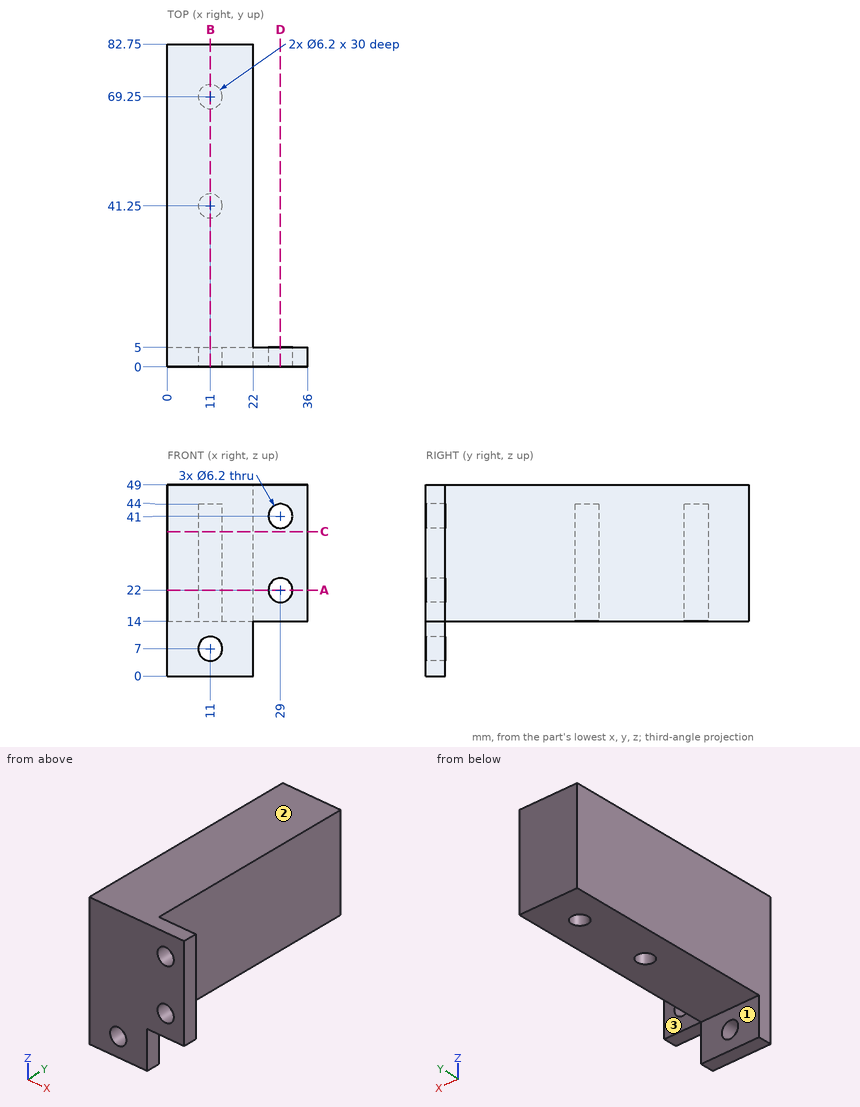
Here's the drawing with two shaded views (mm, measured from the low corner). I have some questions. A direction names the side the tool comes from. Coordinates: 2 decimals unless noted, no trailing zeros. Write each loop counter-clockwise with the first axis right and the second up, starting at its lowest first coordinate (ties: lowest second). Pieces come first, ordered by that corner, then holes. Notation, with made-up numbers: M 14.25,-14.75 L 26.25,-14.75 A28 ccw 26.25,24.25 Z; hole C 54.25,-21.75 d6. An arc over 180 degrees is marked long. Answer as CSV lines item,"result".
Item 1: I'm going to push flat-ended pins straight in: P1, Ø5, axis at y = 66.5, z = 44, coming from the -X side; P2, Ø4, axis at x = 9, z = 6.5, coming from the +Y side; P3, Ø1.5, axis at x = 27, y = 3, coming from the -Z side; P4, Ø2.5, axis at y = 3, z = 4, coming from the +X side. Where does each tip first touch, or does it pass through?
Geometry results:
P1,"stops at x = 0"
P2,"stops at y = 5"
P3,"stops at z = 14"
P4,"stops at x = 22"
Item 2: Please list where these lines run through material, in increasing order: line 1 along Z through (x, y) = (29, 3.3); line 2 along Y through (x, z) = (11, 22); line 3 along X through (y, z) = (69, 36.5).
Geometry results:
line 1,"z = 14 to 18.9, 25.1 to 37.9, 44.1 to 49"
line 2,"y = 0 to 38.15, 44.35 to 66.15, 72.35 to 82.75"
line 3,"x = 0 to 7.91, 14.09 to 22"
Item 3: Imagine slicing it at B-B on x = 11. List the corners of the cut face in (y, z) for me.
Geometry results:
outline,"M 0,0 L 5,0 L 5,3.9 L 0,3.9 Z; M 0,10.1 L 5,10.1 L 5,14 L 38.15,14 L 38.15,44 L 44.35,44 L 44.35,14 L 66.15,14 L 66.15,44 L 72.35,44 L 72.35,14 L 82.75,14 L 82.75,49 L 0,49 Z"
Item 4: Imagine slicing it at A-A on z = 22. List the corners of the cut face in (x, y) for me.
Geometry results:
outline,"M 0,0 L 25.9,0 L 25.9,5 L 22,5 L 22,82.75 L 0,82.75 Z; M 32.1,0 L 36,0 L 36,5 L 32.1,5 Z; hole C 11,41.25 d6.2; hole C 11,69.25 d6.2"
Item 5: Imagine slicing it at C-C on z = 37. List the corners of the cut face in (x, y) for me, plus the area to 3 significant figures.
Geometry results:
outline,"M 0,0 L 36,0 L 36,5 L 22,5 L 22,82.75 L 0,82.75 Z; hole C 11,41.25 d6.2; hole C 11,69.25 d6.2"
area,"1,830 mm2"
Item 6: On a 3-axis mill with a long thin cutter (end or side, diameter ignored), from which of +Z, -Z, +X, -X, +Y, -Y can I reach the whole of each face in a straight line? I mean the marked faces 1, 2 and 3. Say none if no direction works.
Geometry results:
face 1,"-Z, +X, -X, +Y"
face 2,"+Z, +X, -X, +Y, -Y"
face 3,"+Z, -Z, +X, +Y"
Item 7: Imagine slicing it at D-D on x = 29. List the corners of the cut face in (y, z) for me, plus the area to 3 significant figures.
Geometry results:
outline,"M 0,14 L 5,14 L 5,18.9 L 0,18.9 Z; M 0,25.1 L 5,25.1 L 5,37.9 L 0,37.9 Z; M 0,44.1 L 5,44.1 L 5,49 L 0,49 Z"
area,"113 mm2"
